Geometry: final body of the model. Coordinates: model frame, mm. A direction names the side the tool comes from. Give positions to 0.01 mm unless a question says otherwise; leave off trailing zeros. Write each loop counter-clockwise with the first axis right and the second up, starting at its lowest first coordinate (ties: lowest second). Pieces come first, ordered by that corner, then holes. Notation, with made-up numbers: M 20,40 L 68,40 A15 cw 68,64 Z; hole C 71.25,-15 d1. An arc over 180 degrees is marked long. Use one line per item in the form item = value. Start each with the question number.
Item 1: Section query D-D on z = 5. Return loops of the section in (x, y).
Item 2: Section query A-A on z = 0. Return loops of the section in (x, y), then the cut area to 3 significant figures.
Item 3: Pull-direction query (X, two-part tool) for faces 1 (the flat face through (-39.062, 11, 0)), 2 (the cylindrical face through (2.52, 11.34, 6.27)), 3 (the cylindrical face through (6.714, 11.339, -1.283)), 4 (the flat face through (44.339, 11, 0)); classes: released by +X, released by -X, zero draft, split by the parting line, or undercut.
Item 4: Material intervals for line 1 along X through (y, z) = (5.75, 0); line 2 along Z through (x, y) = (-19.5, 7.75); line 3 along X through (y, z) = (19.25, 2.5), sorted ascending. Write a range as from..to.
Item 5: Section query C-C on x = -24. Return loops of the section in (y, z).
Item 6: Contact query for flat-ended pins moving along their axis: P1, Ø1.5, axis at y = 5, z = -2.5, coming from the +X side; P2, Ø2, axis at x = -26, y = 15, coming from the -Z side; P3, Ø1, axis at y = 15, z = 3.5, coming from the +X side; P4, Ø7.5, axis at x = 2.64, z = 0, coming from the -Y side. Output: stop coordinate, or through.
Item 7: Section query B-B on y = 2.5. Return loops of the section in (x, z), then the cut area to 3 significant figures.
Item 8: Access query for faces 5 (the flat face through (-22, 11, -1.542)), 6 (the flat face through (-22, 11, 1.542)), 7 (the flat face through (26, 11, 1.542)). Directions: +Z, -Z, +X, -X, +Y, -Y. A direction counts if a zero-diameter tool reaches every point of the face in a straight line with its end or side. Return the directions, or none.
from build123d import *

# Parameters (mm, degrees)
BOSS_EXTRUDE2_DEPTH      = 23
BOSS_EXTRUDE2_DEPTH_BACK = 0.0001
SKETCH2_R                = 6.272360189
SKETCH2_W                = 83.401872842
SKETCH2_H                = 3.0835427
SHELL3_START             = -0.0001
SHELL3_OUTLINE_R         = 4.272360189
SHELL3_DEPTH             = 23.0001


# Read off the part's stored shape, not the designer's step: Shell3
with BuildPart() as part:
    # Sketch2 → Boss-Extrude2 (new, two sides: drawn at the far end of the back side and taken through both)
    with BuildSketch(Plane(origin=(0, 0, 0), x_dir=(1, 0, 0), z_dir=(0, 1, 0)).offset(-BOSS_EXTRUDE2_DEPTH_BACK)):
        with Locations((2.638515629, 0)):
            Circle(SKETCH2_R)
        with Locations((2.638515629, 0)):
            Rectangle(SKETCH2_W, SKETCH2_H)
    extrude(amount=BOSS_EXTRUDE2_DEPTH + BOSS_EXTRUDE2_DEPTH_BACK)

    # Shell3 outline → Shell3 (cut)
    with BuildSketch(Plane(origin=(0, 0, 0), x_dir=(1, 0, 0), z_dir=(0, 1, 0)).offset(SHELL3_START)):
        with Locations((2.638515629, 0)):
            Circle(SHELL3_OUTLINE_R)
    extrude(amount=SHELL3_DEPTH, mode=Mode.SUBTRACT)


solid = part.part
Answer sheet:
q1.outline = M -1.15,0 L 6.43,0 L 6.43,23 L -1.15,23 Z
q2.outline = M -39.06,0 L -1.63,0 L -1.63,23 L -39.06,23 Z; M 6.91,0 L 44.34,0 L 44.34,23 L 6.91,23 Z
q2.area = 1,720 mm2
q3.face_1 = released by -X
q3.face_2 = split by the parting line
q3.face_3 = undercut
q3.face_4 = released by +X
q4.line_1 = -39.06..-1.63, 6.91..44.34
q4.line_2 = -1.54..1.54
q4.line_3 = -3.11..-0.83, 6.1..8.39
q5.outline = M 0,-1.54 L 23,-1.54 L 23,1.54 L 0,1.54 Z
q6.P1 = 8.66
q6.P2 = -1.54
q6.P3 = 8.15
q6.P4 = through
q7.outline = M -39.06,-1.54 L -3.44,-1.54 A6.27 ccw 8.72,-1.54 L 44.34,-1.54 L 44.34,1.54 L 8.72,1.54 A6.27 ccw -3.44,1.54 L -39.06,1.54 Z; hole C 2.64,0 d8.54
q7.area = 285 mm2
q8.face_5 = -Z, -X, +Y, -Y
q8.face_6 = +Z, -X, +Y, -Y
q8.face_7 = +Z, +X, +Y, -Y
